Can you work these out from the drawing? Everything is in mm from the part's minimum corner. A direction names the side the tool comes from. Give positions to 0.01 mm unless a question says otherwise; leave off trailing zeros. Write each loop counter-clockwise with the first axis right and the second up, starting at its lowest first coordinate (ties: lowest second). Pieces come first, ordered by that corner, then holes. Notation, with made-up numbers: (44, 3.25) - (61, 3.25) arc R16 ccw to (61, 30.25) - close; hole circle Ø10 at (36, -6.5). An arc over 180 degrees is marked (long way). Use a Markdown table: item, result.
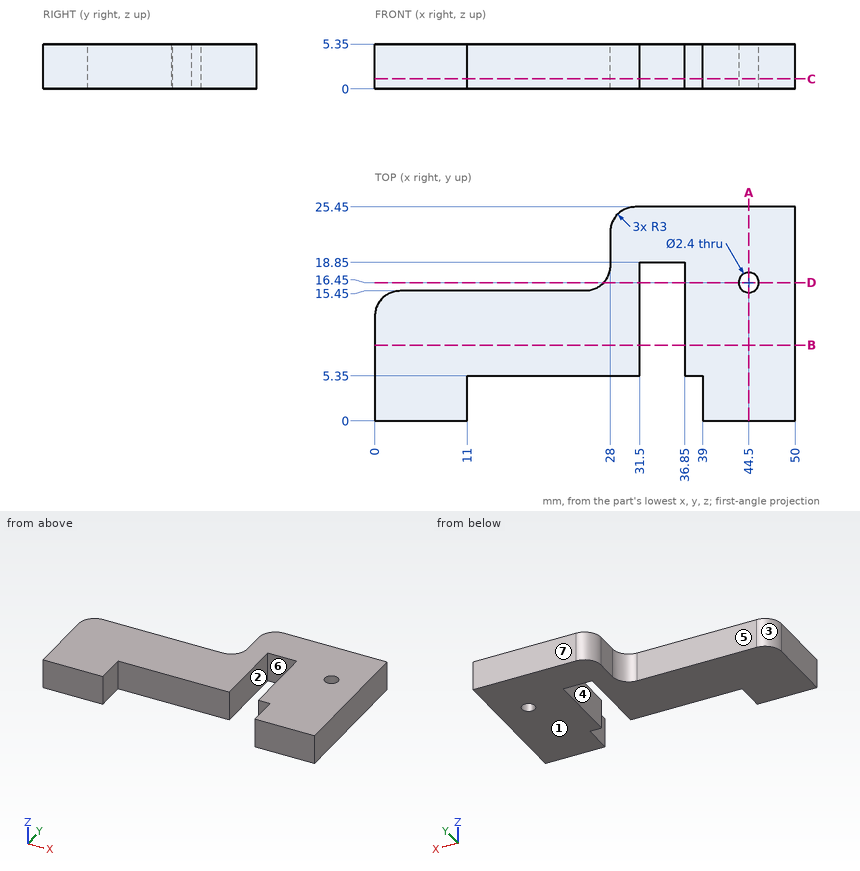
Item 1: If we section it at A-A, the plane x = 44.5: Write out the boundary of the cut face in (y, z).
Values:
| item | result |
|---|---|
| outline | (0, 0) - (15.25, 0) - (15.25, 5.35) - (0, 5.35) - close; (17.65, 0) - (25.45, 0) - (25.45, 5.35) - (17.65, 5.35) - close |
Item 2: For the marked faces 5, 6 and 7, which set-ups out of +Z, -Z, +X, -X, +Y, -Y let a thin tool reach every point of the face, with its end or its side?
Values:
| item | result |
|---|---|
| face 5 | +Z, -Z, -X, +Y |
| face 6 | +Z, -Z, -Y |
| face 7 | +Z, -Z, +X, -X, +Y |
Item 3: If we section it at D-D, the plane y = 16.45: Write out the boundary of the cut face in (x, z).
Values:
| item | result |
|---|---|
| outline | (27.24, 0) - (31.5, 0) - (31.5, 5.35) - (27.24, 5.35) - close; (36.85, 0) - (43.3, 0) - (43.3, 5.35) - (36.85, 5.35) - close; (45.7, 0) - (50, 0) - (50, 5.35) - (45.7, 5.35) - close |
Item 4: Thinking about a two-plate mould opening in X: for the marked faces 1, 2, 3 and 4, which applies, +X half, -X half, draft (parallel to the pull), parting line (faces both ways), or undercut?
Values:
| item | result |
|---|---|
| face 1 | draft |
| face 2 | undercut |
| face 3 | -X half |
| face 4 | undercut |
Item 5: Will these pins go through, and if not, where does the flat tip stop? pin 1 Ø1.1 at (x, z) = (38, 2.5) entering from -Y; pin 2 Ø3 at (y, z) = (21, 2.5) entering from -X; pin 3 Ø2.5 at (x, z) = (34.5, 1.5) entering from -Y.
Values:
| item | result |
|---|---|
| pin 1 | stops at y = 5.35 |
| pin 2 | stops at x = 28 |
| pin 3 | stops at y = 18.85 |
Item 6: I need wall thicknesses on line 1 along X through (y, z) = (7.75, 5.05); line 2 along Y through (x, z) = (44.5, 3); line 3 along X through (y, z) = (16, 0.45). Which ranges of each line are inside material? Lowest first, please. Write a range as [from, to].
Values:
| item | result |
|---|---|
| line 1 | x = [0, 31.5], [36.85, 50] |
| line 2 | y = [0, 15.25], [17.65, 25.45] |
| line 3 | x = [26.73, 31.5], [36.85, 43.39], [45.61, 50] |
Item 7: If we section it at B-B, the plane y = 9: Write out the boundary of the cut face in (x, z).
Values:
| item | result |
|---|---|
| outline | (0, 0) - (31.5, 0) - (31.5, 5.35) - (0, 5.35) - close; (36.85, 0) - (50, 0) - (50, 5.35) - (36.85, 5.35) - close |
Item 8: If we section it at C-C, the plane z = 1.2: Write out the boundary of the cut face in (x, y).
Values:
| item | result |
|---|---|
| outline | (0, 0) - (11, 0) - (11, 5.35) - (31.5, 5.35) - (31.5, 18.85) - (36.85, 18.85) - (36.85, 5.35) - (39, 5.35) - (39, 0) - (50, 0) - (50, 25.45) - (31, 25.45) arc R3 ccw to (28, 22.45) - (28, 18.45) arc R3 cw to (25, 15.45) - (3, 15.45) arc R3 ccw to (0, 12.45) - close; hole circle Ø2.4 at (44.5, 16.45) |
